Could you check a few things on this model? Use its own coordinates, in mm. Face numbers are marked on the shaded views. A direction names the side the tool comes from. Coordinates: 2 decimals unless noted, no trailing zeros. Loops run counter-clockwise (first coordinate to the right, second up) from the corner with the lowest first, then second, coordinate; pieces in that order, holes last.
1) Imagine slicing it at B-B on z = 4. Please give me the cut outline in (x, y), plus the area to 3 significant figures.
2) If I drill on line 1 along Y through (x, z) = (-0.25, -6); line 2 along Y through (x, z) = (0, 5); line 3 along X through (y, z) = (-4, 3.5), over which ranges is the centre line in solid material (lowest first)?
3) Thinking about a two-plate mould opening in X: for the marked faces 1, 2, 3 and 4, which applies, released by +X, released by -X, zero draft, split by the parting line, or undercut?
4) Will these pins go through, and if not, where does the flat tip stop? P1, Ø3, axis at x = 3, z = 1, coming from the -Y side; P2, Ø3.5, axis at y = -1, z = 6.5, coming from the +X side; P3, Ø8, axis at y = 2.5, z = 8, coming from the -X side.
5) Imagine slicing it at C-C on z = -7. Please give me the cut outline in (x, y), plus the area to 3 significant figures.
6) For the marked faces 5, 6 and 7, which set-ups out of +Z, -Z, +X, -X, +Y, -Y let a thin tool reach every point of the face, with its end or its side?
```python
from build123d import *

# Parameters (mm, degrees)
HEAD_DEPTH     = 10
SHANK_SKETCH_R = 6
SHANK_DEPTH    = 30
SKETCH6_R      = 7.875
HEAD_CUT_DEPTH = 1.5
FILLET1_R      = 2
FILLET2_R      = 0.5
THREAD_END_W   = 30
THREAD_END_H   = 0.05


with BuildPart() as part:
    # Head Sketch → Head (new body)
    with BuildSketch(Plane.XY):
        Polygon((0, 10.392304845), (9, 5.196152423), (9, -5.196152423), (0, -10.392304845), (-9, -5.196152423), (-9, 5.196152423), align=None)
    extrude(amount=HEAD_DEPTH)

    # Shank Sketch → Shank (add)
    with BuildSketch(Plane.XY):
        Circle(SHANK_SKETCH_R)
    extrude(amount=-SHANK_DEPTH)

    # Sketch3 → Flange (revolve)
    with BuildSketch(Plane(origin=(0, 0, 0), x_dir=(-1, 0, 0), z_dir=(0, 1, 0)), mode=Mode.PRIVATE) as flange_sk:
        with BuildLine():
            Line((-13, 0), (0, 0))
            Line((0, 0), (0, 5))
            ThreePointArc((0, 5), (-6.947778179, 3.955279081), (-13.281081081, 0.913513514))
            ThreePointArc((-13.281081081, 0.913513514), (-13.477889504, 0.352957076), (-13, 0))
        make_face()
    revolve(flange_sk.sketch.rotate(Axis((0, 0, 0), (0, 0, 1)), 30), axis=Axis((0, 0, 0), (0, 0, 1)))

    # Sketch5 → Head Trim (revolve, cut)
    with BuildSketch(Plane(origin=(0, 0, 0), x_dir=(0, 0, -1), z_dir=(1, 0, 0)), mode=Mode.PRIVATE) as head_trim_sk:
        with BuildLine():
            Line((-10, -8.392304845), (-10, -10.392304845))
            Line((-10, -10.392304845), (-8, -10.392304845))
            ThreePointArc((-8, -10.392304845), (-9.414213562, -9.806518408), (-10, -8.392304845))
        make_face()
    revolve(head_trim_sk.sketch.rotate(Axis((0, 0, 15.085599173), (0, 0, -1)), 90), axis=Axis((0, 0, 15.085599173), (0, 0, -1)), mode=Mode.SUBTRACT)

    # Sketch6 → Head Cut (cut)
    with BuildSketch(Plane.XY.offset(10)):
        Circle(SKETCH6_R)
    extrude(amount=-HEAD_CUT_DEPTH, mode=Mode.SUBTRACT)

    # Fillet1
    # the kernel refuses this fillet: 2 mm, written as the material it adds along each edge
    with BuildSketch(Plane(origin=(0, 0, 8.5), x_dir=(1, 0, 0), z_dir=(0, -1, 0))) as fillet1_piece_1:
        with BuildLine():
            CenterArc((5.938508327, 2), FILLET1_R, 270, 75.522487814)
            Line((5.938508327, 0), (5.938508327, -0.04))
            Line((5.938508327, -0.04), (7.875, -0.04))
            Line((7.875, -0.04), (7.915, 0))
            ThreePointArc((7.915, 0), (7.915, 0.75), (7.913729833, 1.49))
            Line((7.913729833, 1.49), (7.875, 1.5))
        make_face()
    revolve(axis=Axis((0, 0, 8.5), (0, 0, 1)))

    # Fillet2
    fillet2_edges = [part.edges().sort_by_distance(p)[0] for p in [
        (-6, 0, 0),
    ]]
    fillet(fillet2_edges, radius=FILLET2_R)

    # Thread End → Thread Cut (revolve, cut)
    with BuildSketch(Plane(origin=(0, 0, 0), x_dir=(0, 0, -1), z_dir=(1, 0, 0)), mode=Mode.PRIVATE) as thread_cut_sk:
        with Locations((15, 5.975)):
            Rectangle(THREAD_END_W, THREAD_END_H)
    revolve(thread_cut_sk.sketch.rotate(Axis((0, 0, -21.551935625), (0, 0, -1)), 90), axis=Axis((0, 0, -21.551935625), (0, 0, -1)), mode=Mode.SUBTRACT)


solid = part.part
```
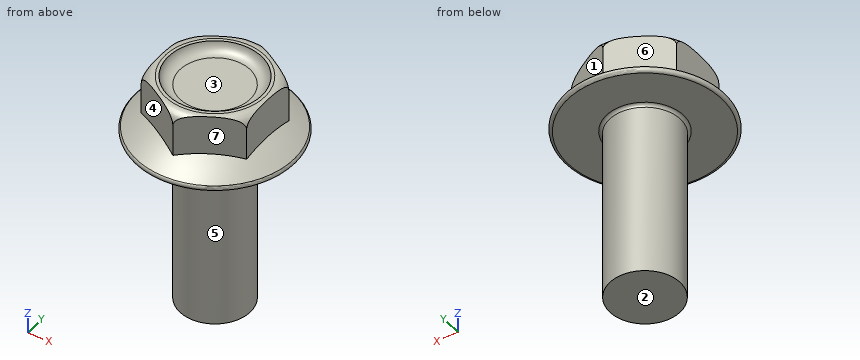
Filled in:
1. outline: (-9, -5.2) - (0, -10.39) - (9, -5.2) - (9, 5.2) - (0, 10.39) - (-9, 5.2) - close
1. area: 281 mm2
2. line 1: y = -5.94 to 5.94
2. line 2: y = -10.39 to 10.39
2. line 3: x = -9 to 9
3. face 1: released by +X
3. face 2: zero draft
3. face 3: undercut
3. face 4: released by -X
4. P1: stops at y = -13.41
4. P2: stops at x = 9
4. P3: stops at x = -9
5. outline: circle Ø11.9 at (0, 0)
5. area: 111 mm2
6. face 5: -Z
6. face 6: +Z, -X, +Y
6. face 7: +Z, +X, -Y
